Geometry check sheet. Reference: drawing and pictorial views, mm from the part's lowest x, y, z. Coordinates: 2 decimals unless noted, no trailing zeros. Write each loop counter-clockwise with the first axis right and the second up, starting at its lowest first coordinate (ties: lowest second). Pieces come first, ordered by that corner, then holes. Notation, with made-up numbers: (58, 84.5) - (104, 84.5) arc R16 ccw to (104, 97.5) - close; hole circle Ø6 at (49, -4.75). An arc over 180 degrees is marked (long way). Use one line per item in the form item = value. Start each with the question number.
(1) Material ranges on line 1 (X direction, y = 1.5, z = 0.5); line 2 (Y direction, x = 3, z = 1.75); line 3 (Z direction, x = 3.75, y = 1.75) (3 decimals), recorded low to high. Write a range as [from, to].
(2) Sectioned sample at A-A (y = 9.25). Record the cut outline in (x, z), and give its area (3 significant figures).
(3) Gauge pin test, flat ends, axial feed: pin 1 Ø0.9 at (x, z) = (4.5, 4.5) entering from -Y; pin 2 Ø1.5 at (x, z) = (5, 2) entering from -Y; pin 3 Ø5 at (y, z) = (18, 1.5) entering from -X; pin 4 Ø3 at (y, z) = (13, 3) entering from +X. Record the tip position at first contact, or that the pin passes through.
(4) Mould release check, pull along X, two halves, no side actions. Record for the marked faces 1, 2, 3 and 4: released by +X, released by -X, zero draft, split by the parting line, or undercut.
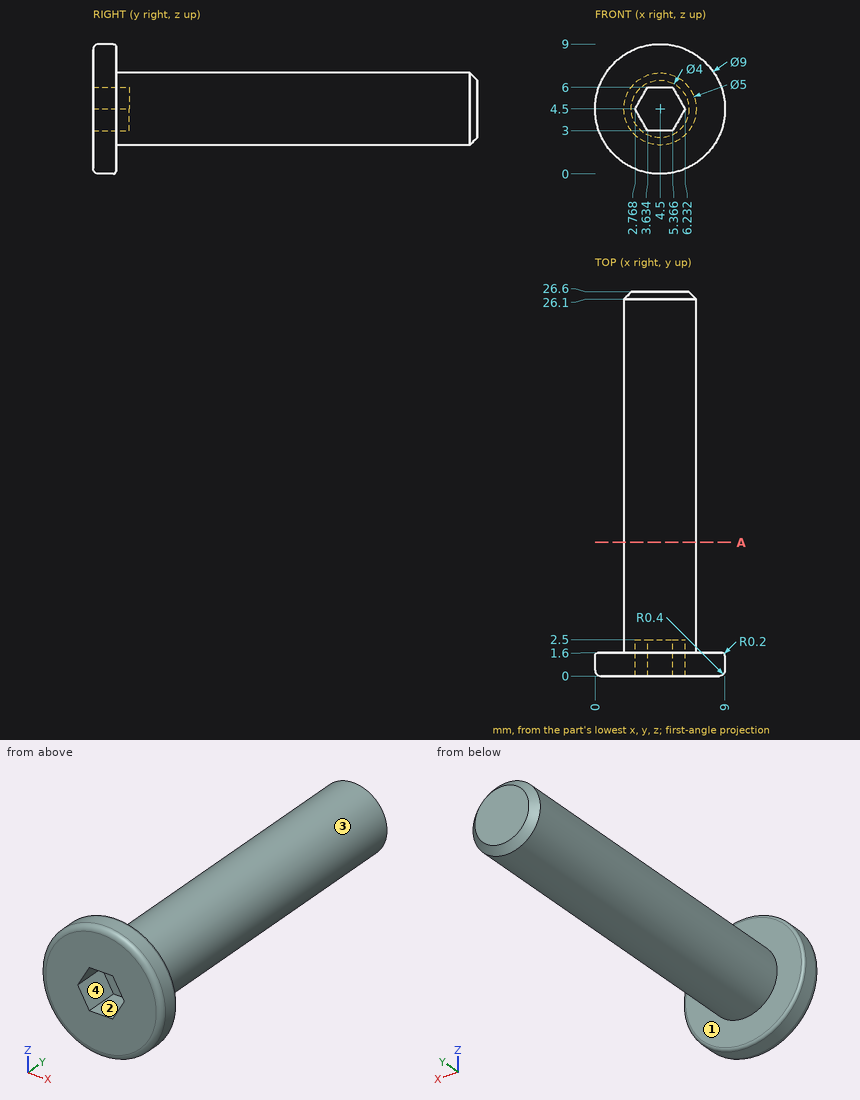
Answers below:
q1.line_1 = [2.5, 6.5]
q1.line_2 = [0, 1.6]
q1.line_3 = [2.115, 3], [6, 6.885]
q2.outline = circle Ø5 at (4.5, 4.5)
q2.area = 19.6 mm2
q3.pin_1 = 2.5
q3.pin_2 = 0
q3.pin_3 = 2.05
q3.pin_4 = 7
q4.face_1 = zero draft
q4.face_2 = undercut
q4.face_3 = split by the parting line
q4.face_4 = undercut
